Work out the finished part from the listing and answer in its coordinate system (mm). Face numbers are marked on the shaded views. Round coordinates to 2 decimals unless told otherwise and drop trailing zeros. Order: outer loops, then holes, each group sorted by start corner. A loop starts at its lowest first (then second) coordinate and runs counter-clockwise, first axis right, second up. Notation, with made-up numbers: (-28.5, -9.5) -> (-3.5, -9.5) arc R26 cw to (-3.5, 15.5) -> close; hole circle Ø9 at (74, 75.25). An arc over 180 degrees is marked (long way). Use one line per item in the form item = value.
```python
from build123d import *

# Parameters (mm, degrees)
SKETCH1_W           = 76.2
SKETCH1_H           = 44.45
BOSS_EXTRUDE1_DEPTH = 5.08
SKETCH4_R           = 15.875
CUT_EXTRUDE2_DEPTH  = 12.7
SKETCH6_W           = 25.4
SKETCH6_H           = 5.08
CUT_EXTRUDE4_DEPTH  = 5.08


with BuildPart() as part:
    # Sketch1 → Boss-Extrude1 (new body)
    with BuildSketch(Plane.XY):
        Rectangle(SKETCH1_W, SKETCH1_H)
    extrude(amount=BOSS_EXTRUDE1_DEPTH)

    # Sketch4 → Cut-Extrude2 (cut)
    with BuildSketch(Plane.XY.offset(5.08)):
        with Locations((0, 4.7625)):
            Circle(SKETCH4_R)
    extrude(amount=-CUT_EXTRUDE2_DEPTH, mode=Mode.SUBTRACT)

    # Sketch6 → Cut-Extrude4 (cut)
    with BuildSketch(Plane.XZ.offset(22.225)):
        with Locations((0, 2.54)):
            Rectangle(SKETCH6_W, SKETCH6_H)
    extrude(amount=-CUT_EXTRUDE4_DEPTH, mode=Mode.SUBTRACT)


solid = part.part
```
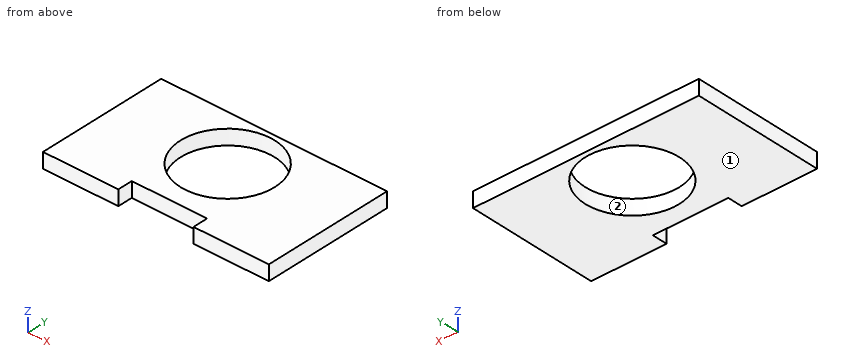
Item 1: Consider line 1 along Y through (x, z) = (0, 3.2) (1 decimal); line 2 along X through (y, z) = (-19.5, 4.6); line 3 along X through (y, z) = (-3, 4.2). Determine where each line is inside the solid, lowest interval first.
Findings:
line_1 = -17.1 to -11.1, 20.6 to 22.2
line_2 = -38.1 to -12.7, 12.7 to 38.1
line_3 = -38.1 to -13.85, 13.85 to 38.1
Item 2: Determine the mould class of the marked faces 1 and 2 for opening direction Y: released by +Y, released by -Y, zero draft, split by the parting line, or undercut.
Findings:
face_1 = zero draft
face_2 = undercut
Item 3: The part is cut by section A-A, the plane x = 0. Give the vertices of the cut face in (y, z) (1 decimal).
Findings:
outline = (-17.1, 0) -> (-11.1, 0) -> (-11.1, 5.1) -> (-17.1, 5.1) -> close; (20.6, 0) -> (22.2, 0) -> (22.2, 5.1) -> (20.6, 5.1) -> close
Item 4: A flat-ended cylindrical pin translates along its axis: P1, Ø1.5, axis at x = 5.5, z = 3, coming from the -Y side (3 decimals). Find the tip coordinate at first contact, or state that the pin passes through.
Findings:
P1 = -17.145
Item 5: The part is cut by section C-C, the plane y = -1. Give the vertices of the cut face in (x, z).
Findings:
outline = (-38.1, 0) -> (-14.79, 0) -> (-14.79, 5.08) -> (-38.1, 5.08) -> close; (14.79, 0) -> (38.1, 0) -> (38.1, 5.08) -> (14.79, 5.08) -> close
